```python
from build123d import *

# Parameters (mm, degrees)
SKETCH1_W           = 176.276
SKETCH1_H           = 25.4
BOSS_EXTRUDE1_DEPTH = 50.8
SKETCH2_OUTSIDE_W   = 64.44
SKETCH2_OUTSIDE_H   = 89.84
SKETCH2_OUTSIDE_W_2 = 25.4
SKETCH2_OUTSIDE_H_2 = 50.8
SKETCH2_OUTSIDE_W_3 = 19.05
SKETCH2_OUTSIDE_H_3 = 44.45
CUT_EXTRUDE1_DEPTH  = 186.199968078
SKETCH3_R           = 14.2875
CUT_EXTRUDE2_DEPTH  = 186.199968078
SKETCH4_R           = 3.3782
CUT_EXTRUDE3_DEPTH  = 186.199968078
SKETCH5_R           = 3.3782
CUT_EXTRUDE4_DEPTH  = 186.199968078


with BuildPart() as part:
    # Sketch1 → Boss-Extrude1 (new body)
    with BuildSketch(Plane(origin=(0, 0, 0), x_dir=(1, 0, 0), z_dir=(0, 1, 0))):
        with Locations((88.138, 12.7)):
            Rectangle(SKETCH1_W, SKETCH1_H)
    extrude(amount=BOSS_EXTRUDE1_DEPTH)

    # Sketch2 outside → Cut-Extrude1 (cut, through all)
    # profile 1 of 2: a face of its own
    with BuildSketch(Plane(origin=(176.276, 0, 0), x_dir=(0, 0, -1), z_dir=(1, 0, 0))):
        with Locations((12.7, 25.4)):
            Rectangle(SKETCH2_OUTSIDE_W, SKETCH2_OUTSIDE_H)
        with Locations((12.7, 25.4)):
            Rectangle(SKETCH2_OUTSIDE_W_2, SKETCH2_OUTSIDE_H_2, mode=Mode.SUBTRACT)
    # profile 2 of 2: a face of its own
    with BuildSketch(Plane(origin=(176.276, 0, 0), x_dir=(0, 0, -1), z_dir=(1, 0, 0))):
        with Locations((12.7, 25.4)):
            Rectangle(SKETCH2_OUTSIDE_W_3, SKETCH2_OUTSIDE_H_3)
    extrude(amount=-CUT_EXTRUDE1_DEPTH, mode=Mode.SUBTRACT)

    # Sketch3 → Cut-Extrude2 (cut, through all)
    with BuildSketch(Plane(origin=(0, 0, -25.4), x_dir=(-1, 0, 0), z_dir=(0, 0, -1))):
        with Locations((-76.2, 25.4)):
            Circle(SKETCH3_R)
    extrude(amount=-CUT_EXTRUDE2_DEPTH, mode=Mode.SUBTRACT)

    # Sketch4 → Cut-Extrude3 (cut, through all)
    with BuildSketch(Plane.XY):
        with Locations((148.336, 38.1)):
            Circle(SKETCH4_R)
        with Locations((129.286, 38.1)):
            Circle(SKETCH4_R)
        with Locations((110.236, 38.1)):
            Circle(SKETCH4_R)
    extrude(amount=-CUT_EXTRUDE3_DEPTH, mode=Mode.SUBTRACT)

    # Sketch5 → Cut-Extrude4 (cut, through all)
    with BuildSketch(Plane.XY):
        with Locations((15.24, 38.1)):
            Circle(SKETCH5_R)
        with Locations((15.24, 12.7)):
            Circle(SKETCH5_R)
        with Locations((34.29, 12.7)):
            Circle(SKETCH5_R)
        with Locations((34.29, 38.1)):
            Circle(SKETCH5_R)
    extrude(amount=-CUT_EXTRUDE4_DEPTH, mode=Mode.SUBTRACT)


solid = part.part
```
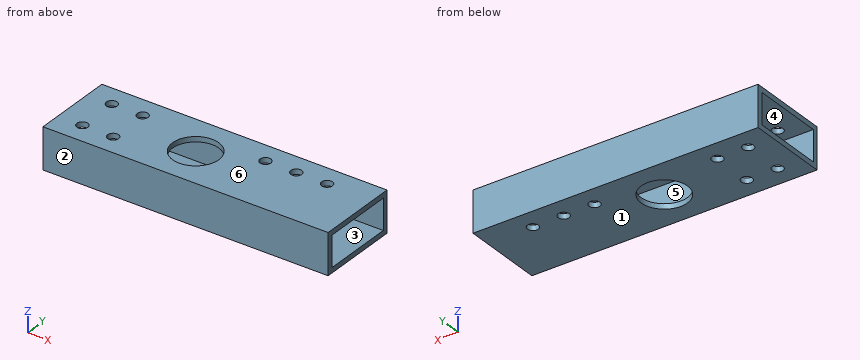
Input: part model. Units: mm. Frame: model coordinates. Face numbers are marked on the shaded views. A direction names the side the tool comes from. Give positions to 0.01 mm unless a question says otherwise; leave off trailing zeros. Order: outer loops, then holes, each group sorted by start corner. A loop starts at its lowest first (then second) coordinate and runs counter-clockwise, first axis right, second up.
1. Draft query along Z for the marked faces 1, 2, 3 and 4. Return one class per face: released by +Z, released by -Z, zero draft, split by the parting line, or undercut.
Computed:
face 1: released by -Z
face 2: zero draft
face 3: undercut
face 4: undercut
2. Cut plane D-D (x = 15.24). Return loops of the section in (y, z) (3 decimals), and give its area (3 significant figures).
Computed:
outline: (0, -25.4) - (9.322, -25.4) - (9.322, -22.225) - (3.175, -22.225) - (3.175, -3.175) - (9.322, -3.175) - (9.322, 0) - (0, 0) - close; (16.078, -25.4) - (34.722, -25.4) - (34.722, -22.225) - (16.078, -22.225) - close; (16.078, -3.175) - (34.722, -3.175) - (34.722, 0) - (16.078, 0) - close; (41.478, -25.4) - (50.8, -25.4) - (50.8, 0) - (41.478, 0) - (41.478, -3.175) - (47.625, -3.175) - (47.625, -22.225) - (41.478, -22.225) - close
area: 358 mm2
3. Cut plane A-A (x = 76.2). Return loops of the section in (y, z) (1 decimal).
Computed:
outline: (0, -25.4) - (11.1, -25.4) - (11.1, -22.2) - (3.2, -22.2) - (3.2, -3.2) - (11.1, -3.2) - (11.1, 0) - (0, 0) - close; (39.7, -25.4) - (50.8, -25.4) - (50.8, 0) - (39.7, 0) - (39.7, -3.2) - (47.6, -3.2) - (47.6, -22.2) - (39.7, -22.2) - close
4. Line query: probe 1 along Y at (x, z) = (15.24, -24.05); probe 2 along Y at (x, z) = (37, -10) (3 decimals); probe 3 along Z at (x, y) = (105.5, 21) (3 decimals). Output: solid intervals per line, ascending.
Computed:
probe 1: y = 0 to 9.32, 16.08 to 34.72, 41.48 to 50.8
probe 2: y = 0 to 3.175, 47.625 to 50.8
probe 3: z = -25.4 to -22.225, -3.175 to 0
5. Cut plane C-C (y = 25.4). Return loops of the section in (x, z) (1 decimal), and give its area (3 significant figures).
Computed:
outline: (0, -25.4) - (61.9, -25.4) - (61.9, -22.2) - (0, -22.2) - close; (0, -3.2) - (61.9, -3.2) - (61.9, 0) - (0, 0) - close; (90.5, -25.4) - (176.3, -25.4) - (176.3, -22.2) - (90.5, -22.2) - close; (90.5, -3.2) - (176.3, -3.2) - (176.3, 0) - (90.5, 0) - close
area: 938 mm2
6. Set-up query: the marked faces 5 and 6. Return all of +Z, -Z, +X, -X, +Y, -Y with unobstructed straight access to the full face (end or side cutting, diameter ignored); none if empty.
Computed:
face 5: +X, -X
face 6: +Z, +X, -X, +Y, -Y
7. Cut plane B-B (z = -5.75). Return loops of the section in (x, y) (3 decimals).
Computed:
outline: (0, 0) - (176.276, 0) - (176.276, 3.175) - (0, 3.175) - close; (0, 47.625) - (176.276, 47.625) - (176.276, 50.8) - (0, 50.8) - close
